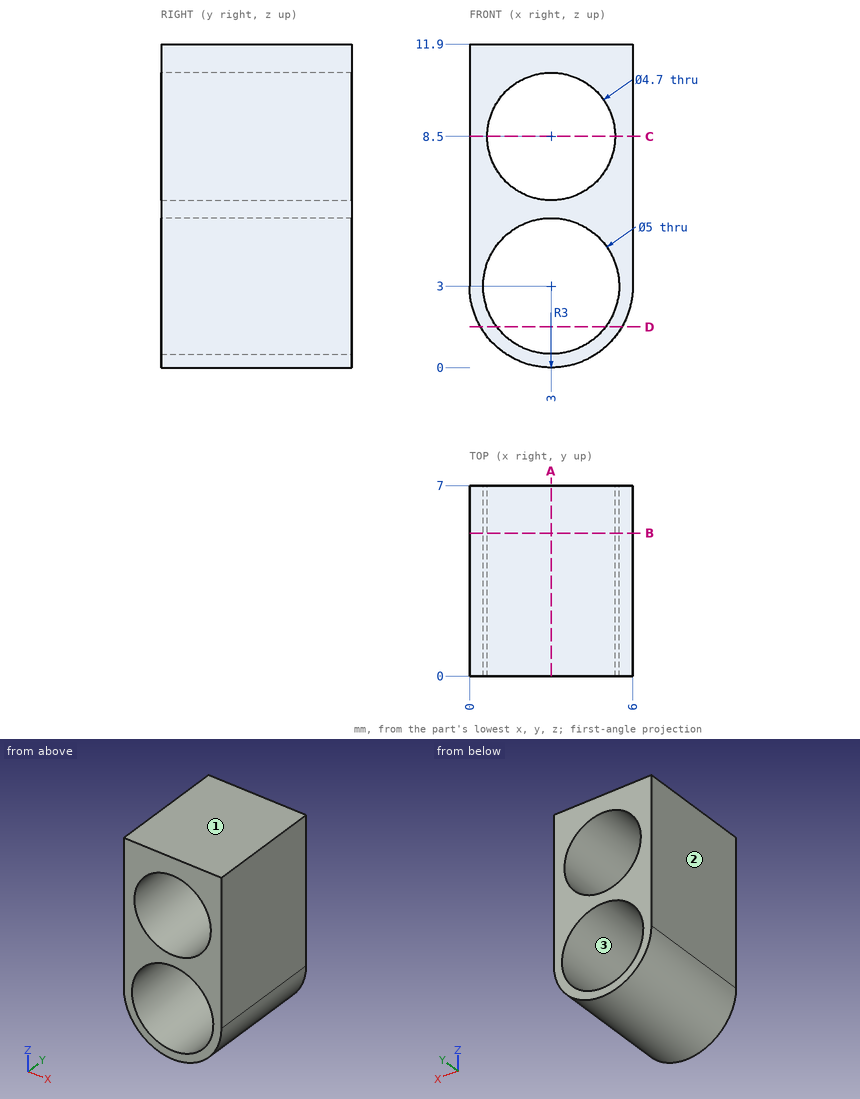
Verification items for this drawing (mm, ordinates from the low corner). Coordinates: 2 decimals unless noted, no trailing zeros. Order: outer loops, then holes, each group sorted by start corner. A loop starts at its lowest first (then second) coordinate and runs counter-clockwise, first axis right, second up.
Q1. Sectioned sample at B-B on y = 5.25. Record the cut outline in (x, z), and give its area (3 significant figures).
Reply:
outline: (0, 3) arc R3 ccw to (6, 3) - (6, 11.9) - (0, 11.9) - close; hole circle Ø5 at (3, 3); hole circle Ø4.7 at (3, 8.5)
area: 30.6 mm2
Q2. Sectioned sample at D-D on z = 1.5. Record the cut outline in (x, y).
Reply:
outline: (0.4, 0) - (1, 0) - (1, 7) - (0.4, 7) - close; (5, 0) - (5.6, 0) - (5.6, 7) - (5, 7) - close
Q3. Sectioned sample at C-C on z = 8.5. Record the cut outline in (x, y).
Reply:
outline: (0, 0) - (0.65, 0) - (0.65, 7) - (0, 7) - close; (5.35, 0) - (6, 0) - (6, 7) - (5.35, 7) - close
Q4. Draft check along Z on the marked faces 1, 2 and 3. Enter one of: released by +Z, released by -Z, zero draft, split by the parting line, or undercut.
Reply:
face 1: released by +Z
face 2: zero draft
face 3: undercut
Q5. Thickness scan on probe 1 along Z at (x, y) = (3.05, 5.75); probe 2 along Z at (x, y) = (5.05, 1.25); probe 3 along X at (y, z) = (6.5, 10). Record the ranges inside material, lowest first.
Reply:
probe 1: z = 0 to 0.5, 5.5 to 6.15, 10.85 to 11.9
probe 2: z = 0.81 to 1.57, 4.43 to 7.35, 9.65 to 11.9
probe 3: x = 0 to 1.19, 4.81 to 6
Q6. Sectioned sample at A-A on x = 3. Record the cut outline in (y, z), and give its area (3 significant figures).
Reply:
outline: (0, 0) - (7, 0) - (7, 0.5) - (0, 0.5) - close; (0, 5.5) - (7, 5.5) - (7, 6.15) - (0, 6.15) - close; (0, 10.85) - (7, 10.85) - (7, 11.9) - (0, 11.9) - close
area: 15.4 mm2
